Answer from the drawing. Dimensions are ordinates in mm from the lowest x, y and z of the part. A direction names the side the tool comes from. Coordinates: 2 decimals unless noted, no trailing zeros. Write each loop counter-clockwise with the first axis right and the second up, starting at its lowest first coordinate (ties: lowest second). Pieces come first, ordered by that corner, then holes. Notation, with made-up numbers: (89, 77) -> (137, 77) arc R11 cw to (137, 97) -> close; hole circle Ø10 at (49, 25). An arc over 180 degrees is marked (long way). Use CSV: the item, a comma, the result in double quotes.
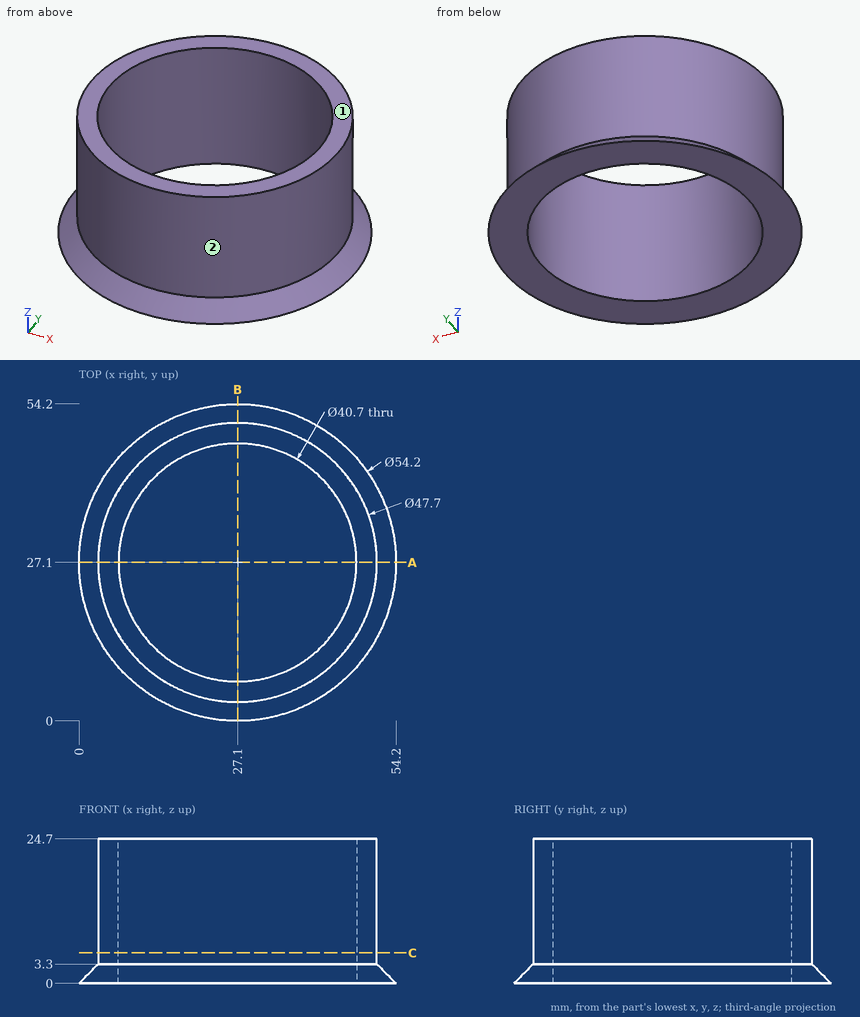
1. A cutting plane is placed at A-A (y = 27.1). Give the vertices of the cut face in (x, z).
Solutions:
outline,"(0, 0) -> (6.75, 0) -> (6.75, 24.7) -> (3.25, 24.7) -> (3.25, 3.3) -> close; (47.45, 0) -> (54.2, 0) -> (50.95, 3.3) -> (50.95, 24.7) -> (47.45, 24.7) -> close"
2. Each of these flat-tipped pins is pushed along its axis until it touches: pin 1 Ø2 at (y, z) = (34, 17) entering from +X; pin 2 Ø4 at (y, z) = (29.5, 14.5) entering from +X; pin 3 Ø3 at (y, z) = (13.5, 13) entering from +X. Where does it stop, or does it pass through?
Solutions:
pin 1,"stops at x = 50.21"
pin 2,"stops at x = 50.95"
pin 3,"stops at x = 47.65"
3. Find the intervals of material crossed by line 1 along X through (y, z) = (27, 9.5); line 2 along X through (y, z) = (15, 19.75), in increasing order.
Solutions:
line 1,"x = 3.25 to 6.75, 47.45 to 50.95"
line 2,"x = 6.55 to 10.74, 43.46 to 47.65"
4. A cutting plane is placed at C-C (z = 5.25). Give the vertices of the cut face in (x, y).
Solutions:
outline,"circle Ø47.7 at (27.1, 27.1); hole circle Ø40.7 at (27.1, 27.1)"
5. A tool of negligible diameter and unlimited length cuts with its end or side. For the marked faces 1 and 2, from which of +Z, -Z, +X, -X, +Y, -Y can it reach the whole face along a straight path? Write none if from no direction.
Solutions:
face 1,"+Z, +X, -X, +Y, -Y"
face 2,"+Z"
